from build123d import *

# Parameters (mm, degrees)
SKETCH_1_R      = 9
SKETCH_1_R_2    = 1.5
EXTRUDE_1_DEPTH = 2.2
CHAMFER_1_SIZE  = 10
FILLET_1_R      = 1.5


with BuildPart() as part:
    # 草图1 → 凸台-拉伸1 (new body)
    with BuildSketch(Plane.XY):
        with BuildLine():
            Line((-17.15, -19.2), (-11.506411256, -19.2))
            ThreePointArc((-11.506411256, -19.2), (0, -26.15), (11.506411256, -19.2))
            Line((11.506411256, -19.2), (17.15, -19.2))
            Line((17.15, -19.2), (17.15, 5.15))
            Line((17.15, 5.15), (-17.15, 5.15))
            Line((-17.15, 5.15), (-17.15, -19.2))
        make_face()
        with BuildLine():
            ThreePointArc((-10.845, -14.195), (-11.139357685, -14.905642315), (-11.85, -15.2))
            Line((-11.85, -15.2), (-14.15, -15.2))
            ThreePointArc((-14.15, -15.2), (-15.155, -14.195), (-14.15, -13.19))
            Line((-14.15, -13.19), (-14.15, -9.01))
            ThreePointArc((-14.15, -9.01), (-15.155, -8.005), (-14.15, -7))
            Line((-14.15, -7), (-11.85, -7))
            ThreePointArc((-11.85, -7), (-11.139357685, -7.294357685), (-10.845, -8.005))
            ThreePointArc((-10.845, -8.005), (-11.139357685, -8.715642315), (-11.85, -9.01))
            Line((-11.85, -9.01), (-11.85, -13.19))
            ThreePointArc((-11.85, -13.19), (-11.139357685, -13.484357685), (-10.845, -14.195))
        make_face(mode=Mode.SUBTRACT)
        with Locations((0, -13.15)):
            Circle(SKETCH_1_R, mode=Mode.SUBTRACT)
        with BuildLine():
            ThreePointArc((11.85, -9.01), (10.845, -8.005), (11.85, -7))
            Line((11.85, -7), (14.15, -7))
            ThreePointArc((14.15, -7), (14.860642315, -7.294357685), (15.155, -8.005))
            ThreePointArc((15.155, -8.005), (14.860642315, -8.715642315), (14.15, -9.01))
            Line((14.15, -9.01), (14.15, -13.19))
            ThreePointArc((14.15, -13.19), (14.860642315, -13.484357685), (15.155, -14.195))
            ThreePointArc((15.155, -14.195), (14.860642315, -14.905642315), (14.15, -15.2))
            Line((14.15, -15.2), (11.85, -15.2))
            ThreePointArc((11.85, -15.2), (10.845, -14.195), (11.85, -13.19))
            Line((11.85, -13.19), (11.85, -9.01))
        make_face(mode=Mode.SUBTRACT)
        with Locations((-7.5, -1.15)):
            Circle(SKETCH_1_R_2, mode=Mode.SUBTRACT)
        with BuildLine():
            Line((2.09, -1.15), (-2.09, -1.15))
            ThreePointArc((-2.09, -1.15), (-3.095, -2.155), (-4.1, -1.15))
            Line((-4.1, -1.15), (-4.1, 1.15))
            ThreePointArc((-4.1, 1.15), (-3.095, 2.155), (-2.09, 1.15))
            Line((-2.09, 1.15), (2.09, 1.15))
            ThreePointArc((2.09, 1.15), (3.095, 2.155), (4.1, 1.15))
            Line((4.1, 1.15), (4.1, -1.15))
            ThreePointArc((4.1, -1.15), (3.095, -2.155), (2.09, -1.15))
        make_face(mode=Mode.SUBTRACT)
        with Locations((7.5, -1.15)):
            Circle(SKETCH_1_R_2, mode=Mode.SUBTRACT)
    extrude(amount=EXTRUDE_1_DEPTH)

    # 倒角1
    chamfer_1_edges = [part.edges().sort_by_distance(p)[0] for p in [
        (-17.15, 5.15, 1.1),
        (17.15, 5.15, 1.1),
    ]]
    chamfer(chamfer_1_edges, length=CHAMFER_1_SIZE)

    # 圆角1
    fillet_1_edges = [part.edges().sort_by_distance(p)[0] for p in [
        (-17.15, -4.85, 1.1),
        (-17.15, -19.2, 1.1),
        (17.15, -19.2, 1.1),
        (11.506411256, -19.2, 1.1),
        (-11.506411256, -19.2, 1.1),
        (-7.15, 5.15, 1.1),
        (7.15, 5.15, 1.1),
        (17.15, -4.85, 1.1),
    ]]
    fillet(fillet_1_edges, radius=FILLET_1_R)


solid = part.part
Work out the finished part from the listing and answer in its coordinate system (mm). A direction names the side the tool comes from. Give positions to 0.01 mm unless a question says otherwise; leave off trailing zeros. Loops run counter-clockwise (first coordinate to the right, second up) from the corner with the lowest first, then second, coordinate; pieces in that order, holes last. Notation, with made-up numbers: (65.5, 1.5) - (107.5, 1.5) arc R20 cw to (107.5, 38.5) - close; hole circle Ø8 at (14.25, 22). An arc over 180 degrees is marked (long way). Answer in a Markdown table with one row per item.
(1) Section A-A (x = 13) is taken. Give the vertices of the cut face in (y, z).
Results list:
| item | result |
|---|---|
| outline | (-19.2, 0) - (-15.2, 0) - (-15.2, 2.2) - (-19.2, 2.2) - close; (-7, 0) - (-0.7, 0) - (-0.7, 2.2) - (-7, 2.2) - close |
(2) Flat-ended cylindrical pins translate along their axes: pin 1 Ø0.7 at (x, z) = (13, 1) entering from -Y; pin 2 Ø0.7 at (x, z) = (-1, 1) entering from -Y; pin 3 Ø0.7 at (y, z) = (0, 0.5) entering from -X. Find the tip coordinate at first contact, or state that the pin passes through.
Results list:
| item | result |
|---|---|
| pin 1 | stops at y = -19.2 |
| pin 2 | stops at y = -26.13 |
| pin 3 | stops at x = -12.65 |
(3) Section D-D (z = 1.8) is taken. State how many separate pieces and enclosed holes the cut face has, and give its area (3 significant figures).
Results list:
| item | result |
|---|---|
| separate pieces | 1 |
| enclosed holes | 6 |
| area | 504 mm² |
(4) For a pull along X with two mould halves and no side action, classify faces 1 (the face through (11.85, -11, 1)), 2 (the face through (0, 5.15, 1)), 3 (the face through (17.15, -12, 1)) as pulls with the +X half, pulls with the -X half, needs draft (parallel to the pull), parting line crosses it, or undercut.
Results list:
| item | result |
|---|---|
| face 1 | undercut |
| face 2 | needs draft |
| face 3 | pulls with the +X half |
(5) Section B-B (x = 0) is taken. Give the vertices of the cut face in (y, z).
Results list:
| item | result |
|---|---|
| outline | (-26.15, 0) - (-22.15, 0) - (-22.15, 2.2) - (-26.15, 2.2) - close; (-4.15, 0) - (-1.15, 0) - (-1.15, 2.2) - (-4.15, 2.2) - close; (1.15, 0) - (5.15, 0) - (5.15, 2.2) - (1.15, 2.2) - close |
(6) Section C-C (y = -8.5) is taken. Give the vertices of the cut face in (x, z).
Results list:
| item | result |
|---|---|
| outline | (-17.15, 0) - (-15.02, 0) - (-15.02, 2.2) - (-17.15, 2.2) - close; (-10.98, 0) - (-7.71, 0) - (-7.71, 2.2) - (-10.98, 2.2) - close; (7.71, 0) - (10.98, 0) - (10.98, 2.2) - (7.71, 2.2) - close; (15.02, 0) - (17.15, 0) - (17.15, 2.2) - (15.02, 2.2) - close |
(7) Consider L1, parallel to Y at x = 7.5, z = 0.7; L2, parallel to Y at x = 14.5, z = 1.2; L3, parallel to X at y = -2, z = 1.2. Determine where each line is inside the solid, lowest interval first. Write a range as [from, to].
Results list:
| item | result |
|---|---|
| L1 | y = [-23.77, -18.12], [-8.18, -2.65], [0.35, 4.79] |
| L2 | y = [-19.2, -15.14], [-13.25, -8.95], [-7.06, -2.2] |
| L3 | x = [-14.3, -8.74], [-6.26, -3.63], [-2.56, 2.56], [3.63, 6.26], [8.74, 14.3] |
(8) A tool of negligible diameter and unlimited length cuts with its end or side. For faces 4 (the face through (-15.155, -8.027, 1.085)), 5 (the face through (0, -3, 2.2)), from which of +Z, -Z, +X, -X, +Y, -Y can it reach the whole face along a straight path? Write none if from no direction.
Results list:
| item | result |
|---|---|
| face 4 | +Z, -Z |
| face 5 | +Z, +X, -X, +Y, -Y |
